```python
from build123d import *

# Parameters (mm, degrees)
SKETCH1_W           = 77
SKETCH1_H           = 64
BOSS_EXTRUDE1_DEPTH = 1.575
SKETCH2_W           = 56
SKETCH2_H           = 30
BOSS_EXTRUDE2_DEPTH = 4
SKETCH3_R           = 3.125
BOSS_EXTRUDE3_DEPTH = 6
SKETCH4_W           = 73
SKETCH4_H           = 55.8
CUT_EXTRUDE1_DEPTH  = 0.1


with BuildPart() as part:
    # Sketch1 → Boss-Extrude1 (new, symmetric)
    with BuildSketch(Plane.XY):
        Rectangle(SKETCH1_W, SKETCH1_H)
    extrude(amount=BOSS_EXTRUDE1_DEPTH, both=True)

    # Sketch2 → Boss-Extrude2 (add)
    with BuildSketch(Plane(origin=(0, 0, -1.575), x_dir=(-1, 0, 0), z_dir=(0, 0, -1))):
        with Locations((-6.5, 8.25)):
            Rectangle(SKETCH2_W, SKETCH2_H)
    extrude(amount=BOSS_EXTRUDE2_DEPTH)

    # Sketch3 → Boss-Extrude3 (add)
    with BuildSketch(Plane(origin=(0, 0, -5.575), x_dir=(-1, 0, 0), z_dir=(0, 0, -1))):
        with Locations((-28.335952563, 18.999270837)):
            Circle(SKETCH3_R)
        with Locations((-17.355937958, 18.999270837)):
            Circle(SKETCH3_R)
        with Locations((-28.335952563, 10.470489708)):
            Circle(SKETCH3_R)
        with BuildLine():
            Line((-6.150306614, 20.999270837), (0.349693386, 20.999270837))
            ThreePointArc((0.349693386, 20.999270837), (2.349693386, 18.999270837), (0.349693386, 16.999270837))
            Line((0.349693386, 16.999270837), (-6.150306614, 16.999270837))
            ThreePointArc((-6.150306614, 16.999270837), (-8.150306614, 18.999270837), (-6.150306614, 20.999270837))
        make_face()
    extrude(amount=BOSS_EXTRUDE3_DEPTH)

    # Sketch4 → Cut-Extrude1 (cut)
    with BuildSketch(Plane.XY.offset(1.575)):
        with Locations((0, 2.1)):
            Rectangle(SKETCH4_W, SKETCH4_H)
    extrude(amount=-CUT_EXTRUDE1_DEPTH, mode=Mode.SUBTRACT)


solid = part.part
```
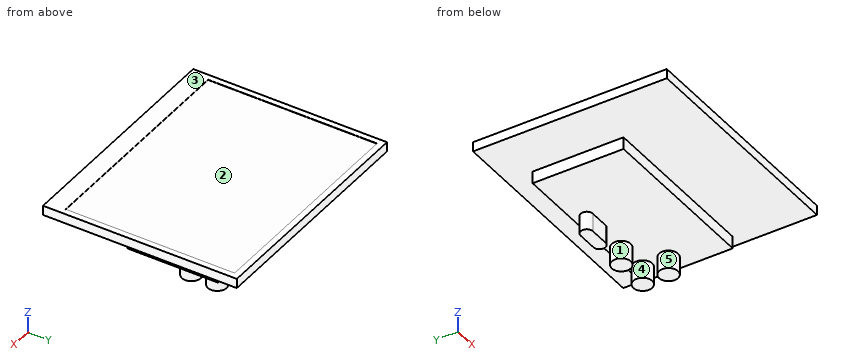
Model file for the job. Use its own axes, mm. Face numbers are marked on the shaded views. A direction names the side the tool comes from. Coordinates: 2 decimals unless noted, no trailing zeros. Write each loop counter-clockwise with the first axis right and the second up, starting at its lowest first coordinate (ties: lowest second). Pieces come first, ordered by that corner, then holes. Notation, with made-up numbers: (-1, 38) - (47, 38) arc R36 ccw to (47, 75) - close; hole circle Ø3 at (8, 79). An arc over 180 degrees is marked (long way). Use a Markdown table: item, result. Add a question column.
Item 1: Band-saw the part on B-B, the plane y = -4.5. Write the cut outline in (x, z) (3 decimals).
Item 2: Two-plate mould, pull along X, no slides. Class the marked faces 3, 4 and 5: pulls with the +X half, pulls with the -X half, needs draft (parallel to the pull), parting line crosses it, or undercut.
Item 3: Drill centre lines: line 1 along X through (y, z) = (20, -9.25); line 2 along Y through (x, z) = (14, -3.5); line 3 along X through (y, z) = (16, -2.5). Where is each one in solid material? Low to high.
Item 4: 3-axis set-ups, long thin cutter, end or side, ignore diameter. For the marked faces 1 and 2: which of +Z, -Z, +X, -X, +Y, -Y reach the whole face in a straight line?
Item 5: Drop flat-ended pins along their axis: pin 1 (3 mm diameter, centred on y = 14, z = -3.5, fed in from -X); pin 2 (1.2 mm diameter, centred on x = 10.5, z = -4, fed in from +Y); pin 3 (1 mm diameter, centred on x = 20.5, y = -3, fed in from -Z) (3 decimals); pin 4 (1.5 mm diameter, centred on y = -11, z = -3.5, fed in from +X). Give the stop position or say it passes through.
Item 6: Band-saw the part on A-A, the plane x = 2. Write the cut outline in (y, z) (3 decimals), and give its area (3 significant figures).
Item 7: Band-saw the part on C-C, the plane z = -9.5. Write the cut outline in (x, y) (3 decimals).
Item 8: Band-saw the part on D-D, the plane y = -22. Write the cut outline in (x, z) (3 decimals).
A:
| question | item | result |
|---|---|---|
| 1 | outline | (-38.5, -1.575) - (-21.5, -1.575) - (-21.5, -5.575) - (34.5, -5.575) - (34.5, -1.575) - (38.5, -1.575) - (38.5, 1.575) - (36.5, 1.575) - (36.5, 1.475) - (-36.5, 1.475) - (-36.5, 1.575) - (-38.5, 1.575) - close |
| 2 | face 3 | needs draft |
| 2 | face 4 | undercut |
| 2 | face 5 | parting line crosses it |
| 3 | line 1 | x = -2.08 to 7.88, 14.4 to 20.32, 25.38 to 31.3 |
| 3 | line 2 | y = -6.75 to 23.25 |
| 3 | line 3 | x = -21.5 to 34.5 |
| 4 | face 1 | -Z |
| 4 | face 2 | +Z |
| 5 | pin 1 | stops at x = -21.5 |
| 5 | pin 2 | stops at y = 23.25 |
| 5 | pin 3 | stops at z = -5.575 |
| 5 | pin 4 | passes through |
| 6 | outline | (-32, -1.575) - (-6.75, -1.575) - (-6.75, -5.575) - (16.999, -5.575) - (16.999, -11.575) - (20.999, -11.575) - (20.999, -5.575) - (23.25, -5.575) - (23.25, -1.575) - (32, -1.575) - (32, 1.575) - (30, 1.575) - (30, 1.475) - (-25.8, 1.475) - (-25.8, 1.575) - (-32, 1.575) - close |
| 6 | area | 340 mm² |
| 7 | outline | (-0.35, 16.999) - (6.15, 16.999) arc R2 ccw to (6.15, 20.999) - (-0.35, 20.999) arc R2 ccw to start; circle Ø6.25 at (17.356, 18.999); circle Ø6.25 at (28.336, 10.47); circle Ø6.25 at (28.336, 18.999) |
| 8 | outline | (-38.5, -1.575) - (38.5, -1.575) - (38.5, 1.575) - (36.5, 1.575) - (36.5, 1.475) - (-36.5, 1.475) - (-36.5, 1.575) - (-38.5, 1.575) - close |
